Work out the finished part from the listing and answer in its coordinate system (mm). A direction names the side the tool comes from. Give positions to 0.01 mm unless a question says otherwise; leave off trailing zeros. Loops run counter-clockwise (first coordinate to the right, second up) from the corner with the lowest first, then second, coordinate; pieces in that order, holes last. Notation, with made-up numbers: M 35.5,-31 L 81.5,-31 A19 cw 81.5,-22 Z; hole C 8.25,-9.75 d3. An arc over 180 degrees is marked long. Answer as a JSON object with one key per item and string values. Group by question number.
```python
from build123d import *

# Parameters (mm, degrees)
SKETCH1_R           = 2.413
BOSS_EXTRUDE1_DEPTH = 13.335
BOSS_EXTRUDE2_DEPTH = 5.08
SKETCH3_R           = 2.413
CUT_EXTRUDE1_DEPTH  = 1.905
SKETCH4_R           = 2.54
BOSS_EXTRUDE3_DEPTH = 2.54
BOSS_EXTRUDE4_DEPTH = 5.08
SKETCH6_R           = 1.5875
BOSS_EXTRUDE5_DEPTH = 5.715
SKETCH7_R           = 2.413
CUT_EXTRUDE2_DEPTH  = 3.175


with BuildPart() as part:
    # Sketch1 → Boss-Extrude1 (new body)
    with BuildSketch(Plane.XY):
        Circle(SKETCH1_R)
    extrude(amount=BOSS_EXTRUDE1_DEPTH)

    # Sketch2 → Boss-Extrude2 (add)
    with BuildSketch(Plane.XY.offset(13.335)):
        Polygon((2.932939367, 0), (1.466469684, 2.54), (-1.466469684, 2.54), (-2.932939367, 0), (-1.466469684, -2.54), (1.466469684, -2.54), align=None)
    extrude(amount=BOSS_EXTRUDE2_DEPTH)

    # Sketch3 → Cut-Extrude1 (cut)
    with BuildSketch(Plane(origin=(0, 0, 0), x_dir=(-1, 0, 0), z_dir=(0, 0, -1))):
        Circle(SKETCH3_R)
    extrude(amount=-CUT_EXTRUDE1_DEPTH, mode=Mode.SUBTRACT)

    # Sketch4 → Boss-Extrude3 (add)
    with BuildSketch(Plane.XY.offset(18.415)):
        with Locations(Location((0, 0, 0), (0, 0, 150))):
            Circle(SKETCH4_R)
    extrude(amount=BOSS_EXTRUDE3_DEPTH)

    # Sketch5 → Boss-Extrude4 (add)
    with BuildSketch(Plane.XY.offset(20.955)):
        Polygon((1.833087105, 0), (0.916543552, 1.5875), (-0.916543552, 1.5875), (-1.833087105, 0), (-0.916543552, -1.5875), (0.916543552, -1.5875), align=None)
    extrude(amount=BOSS_EXTRUDE4_DEPTH)

    # Sketch6 → Boss-Extrude5 (add)
    with BuildSketch(Plane.XY.offset(26.035)):
        with Locations(Location((0, 0, 0), (0, 0, 150))):
            Circle(SKETCH6_R)
    extrude(amount=BOSS_EXTRUDE5_DEPTH)

    # Sketch7 → Cut-Extrude2 (cut)
    with BuildSketch(Plane(origin=(0, 0, 1.905), x_dir=(-1, 0, 0), z_dir=(0, 0, -1))):
        Circle(SKETCH7_R)
    extrude(amount=-CUT_EXTRUDE2_DEPTH, mode=Mode.SUBTRACT)


solid = part.part
```
Item 1: Find the intervals of material crossed by probe 1 along Z at (x, y) = (-1.5, -2.2) (3 decimals); probe 2 along Z at (x, y) = (1.4, 1.5) (3 decimals); probe 3 along Y at (x, z) = (-0.15, 10.5), in increasing order. Write a range as [from, to].
Item 2: A cutting plane is placed at A-A (z = 20). Determine the outline of the cut face in (x, y), and give its area (3 significant figures).
Item 3: Given pin 1 Ø2 at (x, z) = (0, 12) entering from +Y; pin 2 Ø0.6 at (x, y) = (-1.5, 2) entering from +Z (3 decimals); pin 3 Ø0.5 at (x, z) = (0, 23.5) entering from -Y, each flat-ended and moving along its own axis, determine where each tip first touches the part or whether it passes through.
Item 4: A cutting plane is placed at B-B (z = 24.5). Determine the outline of the cut face in (x, y).
Item 5: A tool of negligible diameter and unlimited length cuts with its end or side. For faces 1 (the cylindrical face through (-1.915, -1.468, 9.15)), 2 (the flat face through (1.381, 0.783, 23.459)), 3 (the flat face through (-1.35, -2.33, 18.415)), 4 (the flat face through (1.4, -2.3, 18.415)), from which of +Z, -Z, +X, -X, +Y, -Y can it reach the whole face along a straight path? Write none if from no direction.
Item 6: A cutting plane is placed at C-C (z = 28.75). Determine the outline of the cut face in (x, y) (1 decimal).
The answers:
{
 "1": {"probe 1": "z = [13.335, 18.415]", "probe 2": "z = [5.08, 20.955]", "probe 3": "y = [-2.41, 2.41]"},
 "2": {"outline": "C 0,0 d5.08", "area": "20.3 mm^2"},
 "3": {"pin 1": "stops at y = 2.41", "pin 2": "stops at z = 20.955", "pin 3": "stops at y = -1.59"},
 "4": {"outline": "M -1.83,0 L -0.92,-1.59 L 0.92,-1.59 L 1.83,0 L 0.92,1.59 L -0.92,1.59 Z"},
 "5": {"face 1": "-Z", "face 2": "+Z, +X, +Y", "face 3": "+Z, -X, -Y", "face 4": "+Z, +X, -Y"},
 "6": {"outline": "C 0,0 d3.2"}
}
